Verification items for the finished model (mm, model axes). A direction names the side the tool comes from. Round coordinates to 2 decimals unless told otherwise and drop trailing zeros. Loops run counter-clockwise (first coordinate to the right, second up) from the corner with the lowest first, then second, coordinate; pieces in that order, holes last. Notation, with made-up numbers: (40, 47) - (81, 47) arc R15 cw to (81, 72) - close; hole circle Ø1 at (50, 11). An arc over 180 degrees is marked (long way). Use CSV: the item, a comma, the result in double quotes.
```python
from build123d import *

# Parameters (mm, degrees)
BOX002_W     = 27.49
BOX002_H     = 55
BOX002_DEPTH = 2
BOX_W        = 32.5
BOX_H        = 60
BOX_DEPTH    = 5
FILLET_R     = 1
FILLET001_R  = 1
FILLET002_R  = 1
FILLET003_R  = 1


with BuildPart() as hole_i_frame:
    # Box002 → Box002 (new body)
    with BuildSketch(Plane(origin=(10.1, -51.63, 4), x_dir=(1, 0, 0), z_dir=(0, 0, 1))):
        with Locations((13.745, 27.5)):
            Rectangle(BOX002_W, BOX002_H)
    extrude(amount=BOX002_DEPTH)


with BuildPart() as fillet003:
    # Box → Box (new body)
    with BuildSketch(Plane(origin=(7.6, -54.13, 1), x_dir=(1, 0, 0), z_dir=(0, 0, 1))):
        with Locations((16.25, 30)):
            Rectangle(BOX_W, BOX_H)
    extrude(amount=BOX_DEPTH)

    # Cut: cut Hole i frame
    add(hole_i_frame.part, mode=Mode.SUBTRACT)

    # Fillet
    fillet_edges = [fillet003.edges().sort_by_distance(p)[0] for p in [
        (40.1, 5.87, 3.5),
    ]]
    fillet(fillet_edges, radius=FILLET_R)

    # Fillet001
    fillet001_edges = [fillet003.edges().sort_by_distance(p)[0] for p in [
        (7.6, 5.87, 3.5),
    ]]
    fillet(fillet001_edges, radius=FILLET001_R)

    # Fillet002
    fillet002_edges = [fillet003.edges().sort_by_distance(p)[0] for p in [
        (40.1, -54.13, 3.5),
    ]]
    fillet(fillet002_edges, radius=FILLET002_R)

    # Fillet003
    fillet003_edges = [fillet003.edges().sort_by_distance(p)[0] for p in [
        (7.6, -54.13, 3.5),
    ]]
    fillet(fillet003_edges, radius=FILLET003_R)


with BuildPart() as fillet003_1:
    # Fillet003 placement: moved
    add(fillet003.part.moved(Location((0, 0, 5.5))))


solid = fillet003_1.part
```
1) Cross-section at C-C, the plane x = 18. Record the cut outline in (y, z).
Returned:
outline,"(-54.13, 6.5) - (5.87, 6.5) - (5.87, 11.5) - (3.37, 11.5) - (3.37, 9.5) - (-51.63, 9.5) - (-51.63, 11.5) - (-54.13, 11.5) - close"
2) Thickness scan on probe 1 along Y at (x, z) = (19, 9.6); probe 2 along X at (y, z) = (-41, 9.7); probe 3 along Z at (x, y) = (14, -31.5). Record the ranges inside material, lowest first. Write a range as [from, to].
Returned:
probe 1,"y = [-54.13, -51.63], [3.37, 5.87]"
probe 2,"x = [7.6, 10.1], [37.59, 40.1]"
probe 3,"z = [6.5, 9.5]"
3) Access from +Z, -Z, +X, -X, +Y, -Y to the whole of each face (thin tool, end or side, straight path). Record for faces 5 (the face through (40.1, -25, 9)), 6 (the face through (24, -51.63, 10)).
Returned:
face 5,"+Z, -Z, +X, +Y, -Y"
face 6,"+Z"
4) Gauge pin test, flat end, axial feed: pin 1 Ø2 at (x, y) = (25.5, -24.5) entering from +Z. Record the tip position at first contact, or that the pin passes through.
Returned:
pin 1,"stops at z = 9.5"
5) Cross-section at A-A, the plane z = 10.3. Record the cut outline in (x, y).
Returned:
outline,"(7.6, -53.13) arc R1 ccw to (8.6, -54.13) - (39.1, -54.13) arc R1 ccw to (40.1, -53.13) - (40.1, 4.87) arc R1 ccw to (39.1, 5.87) - (8.6, 5.87) arc R1 ccw to (7.6, 4.87) - close; hole (10.1, -51.63) - (37.59, -51.63) - (37.59, 3.37) - (10.1, 3.37) - close"
6) Mould release check, pull along Y, two halves, no side actions. Record for faces 1 (the face through (24, 5.87, 9)), 2 (the face through (9, -22, 11.5)), 3 (the face through (37.59, -25, 10)), 4 (the face through (10.1, -25, 10)): +Y half, -Y half, draft (parallel to the pull), parting line (faces both ways), or undercut.
Returned:
face 1,"+Y half"
face 2,"draft"
face 3,"undercut"
face 4,"undercut"
7) Cross-section at B-B, the plane y = -19. Record the cut outline in (x, z).
Returned:
outline,"(7.6, 6.5) - (40.1, 6.5) - (40.1, 11.5) - (37.59, 11.5) - (37.59, 9.5) - (10.1, 9.5) - (10.1, 11.5) - (7.6, 11.5) - close"
